Geometry: final body of the model. Coordinates: model frame, mm. Face numbers are marked on the shaded views. A direction names the side the tool comes from. Coordinates: 2 decimals unless noted, no trailing zeros. Loops run counter-clockwise (first coordinate to the right, second up) from the corner with the lowest first, then second, coordinate; pieces in that order, holes last. Notation, with made-up numbers: (-25.5, -4) -> (-16.5, -4) arc R21 cw to (-16.5, 10) -> close; hole circle Ø5 at (67.5, -13.75). An arc over 180 degrees is marked (long way). One line per item, written item: value. Start each with the question number.
from build123d import *

# Parameters (mm, degrees)
SKETCH1_R            = 16.3
BOSS_EXTRUDE1_DEPTH  = 46
SKETCH2_R            = 18.4
BOSS_EXTRUDE2_DEPTH  = 22.1
SKETCH3_R            = 5.9
SKETCH3_R_2          = 2.289263955330087
BOSS_EXTRUDE3_DEPTH  = 5.5
SKETCH4_R            = 2.289263955330087
BOSS_EXTRUDE4_DEPTH  = 35
SKETCH5_R            = 15.4
BOSS_EXTRUDE5_DEPTH  = 0.02
SKETCH7_R            = 1.219257325052135
BOSS_EXTRUDE6_DEPTH  = 4
SKETCH8_R            = 6.650000000000001
BOSS_EXTRUDE7_DEPTH  = 4
BOSS_EXTRUDE9_DEPTH  = 6.5
FILLET3_R            = 0.5
FILLET4_R            = 0.5
BOSS_EXTRUDE10_DEPTH = 5


with BuildPart() as part:
    # Sketch1 → Boss-Extrude1 (new body)
    with BuildSketch(Plane.XY):
        Circle(SKETCH1_R)
    extrude(amount=BOSS_EXTRUDE1_DEPTH)

    # Sketch2 → Boss-Extrude2 (add)
    with BuildSketch(Plane(origin=(0, 0, 0), x_dir=(-1, 0, 0), z_dir=(0, 0, -1))):
        Circle(SKETCH2_R)
    extrude(amount=-BOSS_EXTRUDE2_DEPTH)

    # Sketch3 → Boss-Extrude3 (add)
    with BuildSketch(Plane(origin=(0, 0, 0), x_dir=(-1, 0, 0), z_dir=(0, 0, -1))):
        with Locations(Location((3.05e-15, -6.499999999999999, 0), (0, 0, 180))):
            Circle(SKETCH3_R)
        with Locations((3.05e-15, -6.499999999999999)):
            Circle(SKETCH3_R_2, mode=Mode.SUBTRACT)
    extrude(amount=BOSS_EXTRUDE3_DEPTH)

    # Sketch4 → Boss-Extrude4 (add)
    with BuildSketch(Plane(origin=(0, 0, 0), x_dir=(-1, 0, 0), z_dir=(0, 0, -1))):
        with Locations((3.05e-15, -6.499999999999999)):
            Circle(SKETCH4_R)
    extrude(amount=BOSS_EXTRUDE4_DEPTH)

    # Sketch5 → Boss-Extrude5 (add)
    with BuildSketch(Plane(origin=(0, 0, 0), x_dir=(-1, 0, 0), z_dir=(0, 0, -1))):
        with Locations(Location((0, 0, 0), (0, 0, 180))):
            Circle(SKETCH5_R)
    extrude(amount=BOSS_EXTRUDE5_DEPTH)

    # Sketch7 → Boss-Extrude6 (add)
    with BuildSketch(Plane.XY.offset(46)):
        Circle(SKETCH7_R)
    extrude(amount=BOSS_EXTRUDE6_DEPTH)

    # Sketch8 → Boss-Extrude7 (add)
    with BuildSketch(Plane.XY.offset(50)):
        Circle(SKETCH8_R)
    extrude(amount=BOSS_EXTRUDE7_DEPTH)

    # Sketch9 → Boss-Extrude9 (add)
    with BuildSketch(Plane.XY.offset(46)):
        Polygon((6.723733828483781, -14.005985299746056), (-6.848294391516219, -13.347034241416539), (-6.581571792597097, -7.853505406939939), (6.990456427402904, -8.512456465269457), align=None)
    extrude(amount=BOSS_EXTRUDE9_DEPTH)

    # Fillet3
    fillet3_edges = [part.edges().sort_by_distance(p)[0] for p in [
        (-6.848294391516219, -13.347034241416539, 49.25),
        (-6.714933092056658, -10.60026982417824, 52.5),
        (-0.06228028151621867, -13.676509770581298, 52.5),
    ]]
    fillet(fillet3_edges, radius=FILLET3_R)

    # Fillet4
    fillet4_edges = [part.edges().sort_by_distance(p)[0] for p in [
        (6.723733828483781, -14.005985299746056, 49),
        (6.869218882439666, -11.009515026395185, 52.5),
        (6.730835759440846, -13.859710995839299, 52.35355339059328),
    ]]
    fillet(fillet4_edges, radius=FILLET4_R)

    # Sketch10 → Boss-Extrude10 (add)
    with BuildSketch(Plane.XY.offset(46)):
        with BuildLine():
            Line((-13.903663432832225, 1.1177381723245752), (-13.903663432832225, -1.3957121223426263))
            ThreePointArc((-13.903663432832225, -1.3957121223426263), (-13.757216823425498, -1.7492655129359036), (-13.403663432832222, -1.8957121223426299))
            Line((-13.403663432832222, -1.8957121223426299), (-12.829664566070878, -1.8957121223426299))
            ThreePointArc((-12.829664566070878, -1.8957121223426299), (-12.476111175477602, -1.7492655129359036), (-12.329664566070875, -1.3957121223426263))
            Line((-12.329664566070875, -1.3957121223426263), (-12.329664566070875, 1.1177381723245752))
            ThreePointArc((-12.329664566070875, 1.1177381723245752), (-12.476111175477602, 1.4712915629178525), (-12.829664566070878, 1.6177381723245787))
            Line((-12.829664566070878, 1.6177381723245787), (-13.403663432832222, 1.6177381723245787))
            ThreePointArc((-13.403663432832222, 1.6177381723245787), (-13.757216823425498, 1.4712915629178525), (-13.903663432832225, 1.1177381723245752))
        make_face()
        with BuildLine():
            Line((13.403663432832222, -1.8957121223426299), (12.829664566070878, -1.8957121223426299))
            ThreePointArc((12.829664566070878, -1.8957121223426299), (12.476111175477602, -1.7492655129359036), (12.329664566070875, -1.3957121223426263))
            Line((12.329664566070875, -1.3957121223426263), (12.329664566070875, 1.1177381723245752))
            ThreePointArc((12.329664566070875, 1.1177381723245752), (12.476111175477602, 1.4712915629178525), (12.829664566070878, 1.6177381723245787))
            Line((12.829664566070878, 1.6177381723245787), (13.403663432832222, 1.6177381723245787))
            ThreePointArc((13.403663432832222, 1.6177381723245787), (13.757216823425498, 1.4712915629178525), (13.903663432832225, 1.1177381723245752))
            Line((13.903663432832225, 1.1177381723245752), (13.903663432832225, -1.3957121223426263))
            ThreePointArc((13.903663432832225, -1.3957121223426263), (13.757216823425498, -1.7492655129359036), (13.403663432832222, -1.8957121223426299))
        make_face()
    extrude(amount=BOSS_EXTRUDE10_DEPTH)


solid = part.part
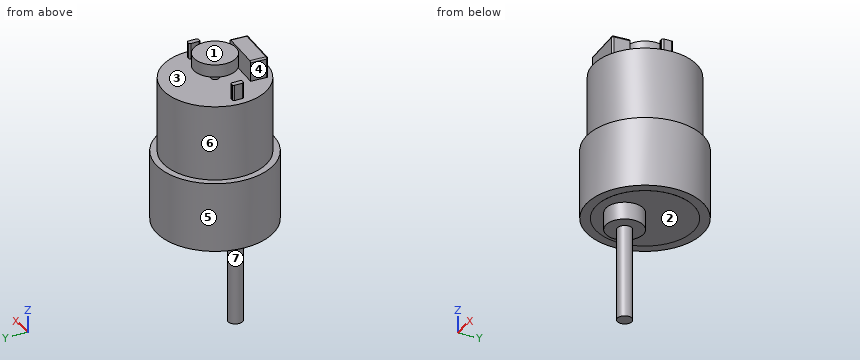
1. Pin query (flat end, axial travel): pin 1 Ø12 at (y, z) = (8.5, 41.5) entering from +X; pin 2 Ø0.8 at (x, y) = (-13, -0.5) entering from +Z; pin 3 Ø4 at (x, y) = (3, -2.5) entering from -Z. Return the tip coordinate at first contact, or that it passes through.
2. Draft query along Z for the marked faces 1, 2, 3 and 4. Return one class per face: released by +Z, released by -Z, zero draft, split by the parting line, or undercut.
3. Section D-D on z = -4.5. Return the cut outline in (x, y), plus the area to 3 significant figures.
4. Set-up query: the marked faces 5, 6 and 7. Return all of +Z, -Z, +X, -X, +Y, -Y with unobstructed straight access to the full face (end or side cutting, diameter ignored); none if empty.
5. Section A-A on z = -20. Return the cut outline in (x, y), plus the area to 3 significant figures.
6. Line query: L1, parallel to Z at x = 2.5, y = -5.5; L2, parallel to Z at x = 0.5, y = 2; L3, parallel to Z at x = -10, y = -2. Output: solid intervals per line, ascending. Write a range as [from, to].
Checks:
1. pin 1: x = 16.11
1. pin 2: z = 51
1. pin 3: z = -5.5
2. face 1: released by +Z
2. face 2: released by -Z
2. face 3: undercut
2. face 4: zero draft
3. outline: circle Ø11.8 at (0, -6.5)
3. area: 109 mm²
4. face 5: +Z, -Z
4. face 6: +Z
4. face 7: -Z
5. outline: circle Ø4.58 at (0, -6.5)
5. area: 16.5 mm²
6. L1: [-5.5, 46], [50, 54]
6. L2: [-0.02, 46], [50, 54]
6. L3: [-0.02, 46]
